```python
from build123d import *

# Parameters (mm, degrees)
ESBO_O1_R                = 1.5
ESBO_O1_R_2              = 5.85
ESBO_O1_W                = 3
ESBO_O1_H                = 10
ESBO_O1_W_2              = 8
ESBO_O1_H_2              = 3
ESBO_O1_W_3              = 15.25
ESBO_O1_H_3              = 5.7
ESBO_O1_W_4              = 18.7
ESBO_O1_H_4              = 12.1
RESSALTO_EXTRUS_O1_DEPTH = 3


with BuildPart() as part:
    # Esboço1 → Ressalto-extrusão1 (new body)
    with BuildSketch(Plane(origin=(0, 0, 0), x_dir=(1, 0, 0), z_dir=(0, 1, 0))):
        with BuildLine():
            Line((110.386890532, 33), (113.308680045, 33))
            ThreePointArc((113.308680045, 33), (128.61601734, 36.0448187), (141.592951292, 44.715728753))
            Line((141.592951292, 44.715728753), (158.868600568, 61.991378029))
            ThreePointArc((158.868600568, 61.991378029), (172.303629411, 58.455844123), (175.839163317, 45.02081528))
            Line((175.839163317, 45.02081528), (158.563514041, 27.745166004))
            ThreePointArc((158.563514041, 27.745166004), (149.892603988, 14.768232051), (146.847785288, -0.539105243))
            Line((146.847785288, -0.539105243), (146.847785288, -3.460894757))
            ThreePointArc((146.847785288, -3.460894757), (149.892603988, -18.768232051), (158.563514041, -31.745166004))
            Line((158.563514041, -31.745166004), (175.839163317, -49.02081528))
            ThreePointArc((175.839163317, -49.02081528), (172.303629411, -62.455844123), (158.868600568, -65.991378029))
            Line((158.868600568, -65.991378029), (141.592951292, -48.715728753))
            ThreePointArc((141.592951292, -48.715728753), (128.61601734, -40.0448187), (113.308680045, -37))
            Line((113.308680045, -37), (110.386890532, -37))
            ThreePointArc((110.386890532, -37), (95.079553237, -40.0448187), (82.102619284, -48.715728753))
            Line((82.102619284, -48.715728753), (64.826970008, -65.991378029))
            ThreePointArc((64.826970008, -65.991378029), (51.391941166, -62.455844123), (47.85640726, -49.02081528))
            Line((47.85640726, -49.02081528), (65.132056536, -31.745166004))
            ThreePointArc((65.132056536, -31.745166004), (73.802966589, -18.768232051), (76.847785288, -3.460894757))
            Line((76.847785288, -3.460894757), (76.847785288, -0.539105243))
            ThreePointArc((76.847785288, -0.539105243), (73.802966589, 14.768232051), (65.132056536, 27.745166004))
            Line((65.132056536, 27.745166004), (47.85640726, 45.02081528))
            ThreePointArc((47.85640726, 45.02081528), (51.391941166, 58.455844123), (64.826970008, 61.991378029))
            Line((64.826970008, 61.991378029), (82.102619284, 44.715728753))
            ThreePointArc((82.102619284, 44.715728753), (95.079553237, 36.0448187), (110.386890532, 33))
        make_face()
        with Locations(Location((111.847785288, 27, 0), (0, 0, 270))):
            Circle(ESBO_O1_R, mode=Mode.SUBTRACT)
        with Locations(Location((111.847785288, -31, 0), (0, 0, 270))):
            Circle(ESBO_O1_R, mode=Mode.SUBTRACT)
        with Locations(Location((169.828664477, -59.980879188, 0), (0, 0, 270))):
            Circle(ESBO_O1_R, mode=Mode.SUBTRACT)
        with Locations(Location((148.615552241, -38.767766953, 0), (0, 0, 270))):
            Circle(ESBO_O1_R, mode=Mode.SUBTRACT)
        with Locations(Location((148.615552241, 34.767766953, 0), (0, 0, 270))):
            Circle(ESBO_O1_R, mode=Mode.SUBTRACT)
        with Locations(Location((169.828664477, 55.980879188, 0), (0, 0, 270))):
            Circle(ESBO_O1_R, mode=Mode.SUBTRACT)
        with Locations(Location((75.080018335, 34.767766953, 0), (0, 0, 270))):
            Circle(ESBO_O1_R, mode=Mode.SUBTRACT)
        with Locations(Location((53.8669061, 55.980879188, 0), (0, 0, 270))):
            Circle(ESBO_O1_R, mode=Mode.SUBTRACT)
        with Locations(Location((117.347785288, 7.1, 0), (0, 0, 270))):
            Circle(ESBO_O1_R, mode=Mode.SUBTRACT)
        with Locations(Location((53.8669061, -59.980879188, 0), (0, 0, 270))):
            Circle(ESBO_O1_R, mode=Mode.SUBTRACT)
        with Locations(Location((75.080018335, -38.767766953, 0), (0, 0, 270))):
            Circle(ESBO_O1_R, mode=Mode.SUBTRACT)
        with Locations(Location((117.347785288, -9, 0), (0, 0, 270))):
            Circle(ESBO_O1_R, mode=Mode.SUBTRACT)
        with Locations(Location((83.347785288, 8, 0), (0, 0, 270))):
            Circle(ESBO_O1_R, mode=Mode.SUBTRACT)
        with Locations(Location((83.347785288, -12, 0), (0, 0, 270))):
            Circle(ESBO_O1_R, mode=Mode.SUBTRACT)
        with Locations(Location((140.347785288, 8, 0), (0, 0, 270))):
            Circle(ESBO_O1_R, mode=Mode.SUBTRACT)
        with Locations(Location((140.347785288, -12, 0), (0, 0, 270))):
            Circle(ESBO_O1_R, mode=Mode.SUBTRACT)
        with Locations(Location((141.592951292, -31, 0), (0, 0, 270))):
            Circle(ESBO_O1_R_2, mode=Mode.SUBTRACT)
        with Locations((83.347785288, -2)):
            Rectangle(ESBO_O1_W, ESBO_O1_H, mode=Mode.SUBTRACT)
        with Locations((125.847785288, -31)):
            Rectangle(ESBO_O1_W_2, ESBO_O1_H_2, mode=Mode.SUBTRACT)
        with Locations((140.347785288, -2)):
            Rectangle(ESBO_O1_W, ESBO_O1_H, mode=Mode.SUBTRACT)
        with Locations((97.847785288, -31)):
            Rectangle(ESBO_O1_W_2, ESBO_O1_H_2, mode=Mode.SUBTRACT)
        with Locations((97.847785288, 27)):
            Rectangle(ESBO_O1_W_2, ESBO_O1_H_2, mode=Mode.SUBTRACT)
        with Locations((98.722785288, 20.094707965)):
            Rectangle(ESBO_O1_W_3, ESBO_O1_H_3, mode=Mode.SUBTRACT)
        with Locations((125.847785288, 27)):
            Rectangle(ESBO_O1_W_2, ESBO_O1_H_2, mode=Mode.SUBTRACT)
        with Locations((121.197785288, 16.894707965)):
            Rectangle(ESBO_O1_W_4, ESBO_O1_H_4, mode=Mode.SUBTRACT)
        Polygon((165.603972833, -59.256005764), (169.121648896, -55.738329701), (171.59652263, -53.263455967), (163.464794646, -45.131727984), (155.333066663, -37), (146.847785288, -45.485281374), (163.111241256, -61.748737342), align=None, mode=Mode.SUBTRACT)
        Polygon((163.464794646, 41.131727984), (155.333066663, 33), (146.847785288, 41.485281374), (163.111241256, 57.748737342), (165.603972833, 55.256005764), (169.121648896, 51.738329701), (171.59652263, 49.263455967), align=None, mode=Mode.SUBTRACT)
        Polygon((104.847785288, 8.6), (104.847785288, -10.5), (106.347785288, -10.5), (106.347785288, 7.873666298), (106.347785288, 8.6), align=None, mode=Mode.SUBTRACT)
        Polygon((68.716057305, 49.617009358), (76.847785288, 41.485281374), (68.362503914, 33), (52.099047947, 49.263455967), (54.591779524, 51.756187545), (58.109455587, 55.273863607), (60.584329321, 57.748737342), align=None, mode=Mode.SUBTRACT)
        Polygon((54.591779524, -55.756187545), (58.109455587, -59.273863607), (60.584329321, -61.748737342), (68.716057305, -53.617009358), (76.847785288, -45.485281374), (68.362503914, -37), (52.099047947, -53.263455967), align=None, mode=Mode.SUBTRACT)
    extrude(amount=RESSALTO_EXTRUS_O1_DEPTH)


solid = part.part
```
Part model, mm, in its own coordinate system. A direction names the side the tool comes from. Round coordinates to 2 decimals unless told otherwise and drop trailing zeros. Loops run counter-clockwise (first coordinate to the right, second up) from the corner with the lowest first, then second, coordinate; pieces in that order, holes last. Notation, with made-up numbers: (89, -14.75) -> (112, -14.75) arc R22 ccw to (112, 24.25) -> close; hole circle Ø6 at (69, 27). An arc over 180 degrees is marked (long way). Use CSV: the item, a comma, the result in double quotes. Start each with the question number.
1) Drop flat-ended pins along their axis: P1, Ø0.9, axis at x = 96.5, y = 1.5, coming from the +Z side; P2, Ø1.5, axis at x = 122.5, y = 2.5, coming from the +Z side; P3, Ø1.5, axis at x = 141, y = 2, coming from the -Z side. Give the stop position or say it passes through.
2) Cut at A-A, the plane z = -21. Write the cut outline in (x, y), plus the area to 3 significant figures.
3) Wall check: L1, parallel to X at y = 2.3, z = 11; L2, parallel to X at y = 0.9, z = 59.5; L3, parallel to Z at x = 58.5, y = 2.1. Give the ranges that are in metal, low to high. Write a range as [from, to].
4) Cut at C-C, the plane y = 2.4. Give the number of separate pieces and of enclosed holes in the cut face, plus the area to 3 significant figures.
5) Cut at B-B, the plane z = 9. Write the cut outline in (x, y).
6) Which spindle directions (+Z, -Z, +X, -X, +Y, -Y) get a long thin tool onto all of the face, cutting with end or side? Do faces 1 (the cylindrical face through (128.82, 1.48, 40.13)), 2 (the flat face through (112, 1, -33)), 3 (the flat face through (91.098, 1, -20)). Say none if no direction does.
Determined:
1,P1,"stops at z = 39.66"
1,P2,"stops at z = 38.26"
1,P3,"stops at z = -44.87"
2,outline,"(70.55, 0) -> (91.1, 0) -> (91.1, 3) -> (70.55, 3) -> close; (106.35, 0) -> (111.85, 0) -> (111.85, 3) -> (106.35, 3) -> close; (130.55, 0) -> (153.14, 0) -> (153.14, 3) -> (130.55, 3) -> close"
2,area,"146 mm2"
3,L1,"x = [76.13, 82.23], [84.47, 139.23], [141.47, 147.56]"
3,L2,"x = [49.14, 52.45], [55.29, 58.34], [62.83, 71.32], [152.38, 160.86], [165.36, 168.41], [171.25, 174.55]"
3,L3,"z = [-62.24, -55.66], [-42.86, -34.38], [38.38, 46.86], [59.66, 66.24]"
4,separate pieces,"1"
4,enclosed holes,"30"
4,area,"7,190 mm2"
5,outline,"(76.46, 0) -> (104.85, 0) -> (104.85, 3) -> (76.46, 3) -> close; (106.35, 0) -> (115.85, 0) -> (115.85, 3) -> (106.35, 3) -> close; (118.85, 0) -> (147.23, 0) -> (147.23, 3) -> (118.85, 3) -> close"
6,face 1,"+Z, +Y, -Y"
6,face 2,"-Z, +Y, -Y"
6,face 3,"+Y, -Y"
